```python
from build123d import *

# Parameters (mm, degrees)
SKETCH1_R           = 4.1
BOSS_EXTRUDE1_DEPTH = 60


with BuildPart() as part:
    # Sketch1 → Boss-Extrude1 (new body)
    with BuildSketch(Plane(origin=(0, 0, 0), x_dir=(0, 0, -1), z_dir=(1, 0, 0))):
        Polygon((0, 0), (-100, 0), (-100, 20), (-31.805308068, 70.001510114), (-22.998489886, 70.001510114), (-13, 80), (0, 80), align=None)
        with Locations((-11.5, 72.5)):
            Circle(SKETCH1_R, mode=Mode.SUBTRACT)
        with Locations((-72.5, 11.5)):
            Circle(SKETCH1_R, mode=Mode.SUBTRACT)
    extrude(amount=BOSS_EXTRUDE1_DEPTH)


solid = part.part
```
The model under review builds one solid part; all positions refer to its coordinate system, in mm. Round coordinates to 2 decimals unless told otherwise and drop trailing zeros. Loops run counter-clockwise (first coordinate to the right, second up) from the corner with the lowest first, then second, coordinate; pieces in that order, holes last. Notation, with made-up numbers: M -9.5,27.25 L 48.5,27.25 A25 cw 48.5,51.25 Z; hole C 16,24.5 d4. An arc over 180 degrees is marked long. Write item = value, one per line.
Item 1: Take a section at B-B on x = 31. Write out the cut boundary in (y, z).
Return value:
outline = M 0,0 L 80,0 L 80,13 L 70,23 L 70,31.81 L 20,100 L 0,100 Z; hole C 11.5,72.5 d8.2; hole C 72.5,11.5 d8.2
Item 2: Insertion check: P1, Ø6, axis at x = 16.5, y = 25.5, coming from the +Z side; P2, Ø9.5, axis at x = 23.5, z = 27, coming from the +Y side; P3, Ø5, axis at x = 16.5, z = 43, coming from the +Y side. Each pin has a flat end and moves straight along its axis. Give the tip position at first contact, or say it passes through.
Return value:
P1 = 96.59
P2 = 70.75
P3 = 63.63
Item 3: For line 1 (Y direction, x = 14, z = 11.5); line 2 (Y direction, x = 45, z = 72.5); line 3 (Z direction, x = 28, y = 11), list the stretches that pass through material, from the lowest coordinate up. Write a range as [from, to].
Return value:
line_1 = [0, 68.4], [76.6, 80]
line_2 = [0, 7.4], [15.6, 40.16]
line_3 = [0, 68.43], [76.57, 100]
Item 4: The part is to be moulded in two halves that separate along Z. For faces 1 (the flat face through (30, 70.002, 27)), 2 (the flat face through (30, 75, 18)), 3 (the flat face through (30, 41, 0)), 4 (the cylindrical face through (29.58, 76.565, 12.034)), say which applies: released by +Z, released by -Z, zero draft, split by the parting line, or undercut.
Return value:
face_1 = zero draft
face_2 = released by +Z
face_3 = released by -Z
face_4 = undercut
Item 5: Take a section at A-A on z = 11.5. Write out the cut boundary in (x, y), then the cut area to 3 significant figures.
Return value:
outline = M 0,0 L 60,0 L 60,68.4 L 0,68.4 Z; M 0,76.6 L 60,76.6 L 60,80 L 0,80 Z
area = 4,310 mm2
Item 6: Take a section at C-C on y = 11.5. Write out the cut boundary in (x, z).
Return value:
outline = M 0,0 L 60,0 L 60,68.4 L 0,68.4 Z; M 0,76.6 L 60,76.6 L 60,100 L 0,100 Z
Item 7: Take a section at D-D on z = 47. Write out the cut boundary in (x, y), then the cut area to 3 significant figures.
Return value:
outline = M 0,0 L 60,0 L 60,58.86 L 0,58.86 Z
area = 3,530 mm2
